Source: CAD feature listing. Evaluate the final solid. Frame: model axes, mm. Face numbers are marked on the shaded views. A direction names the side the tool comes from. Coordinates: 2 decimals unless noted, no trailing zeros. Loops run counter-clockwise (first coordinate to the right, second up) from the corner with the lowest first, then second, coordinate; pieces in that order, holes last. Notation, with made-up numbers: (3, 12.25) - (9, 12.25) arc R20 cw to (9, 39.25) - close; hole circle Ø5 at (50, 7). An arc over 180 degrees is marked (long way). Use CSV: the item, a comma, the result in double quotes. Start each with the question number.
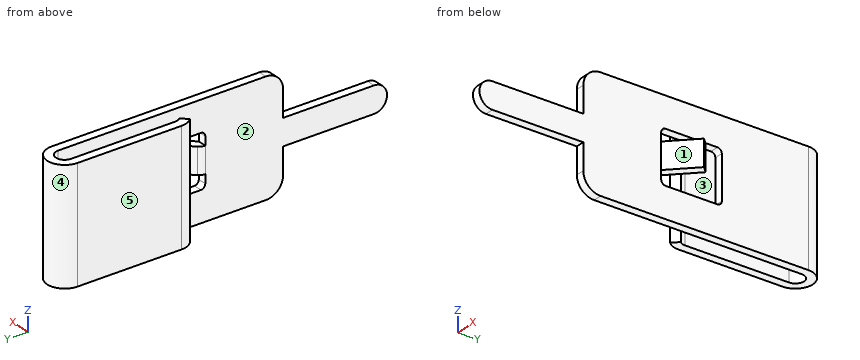
```python
from build123d import *

# Parameters (mm, degrees)
EXTRUDE_1_DEPTH     = 6.5
CUT_EXTRUDE_1_DEPTH = 2
SKETCH_3_W          = 2
SKETCH_3_H          = 2
CUT_EXTRUDE_2_DEPTH = 2.5
SKETCH_4_W          = 2
SKETCH_4_H          = 2
CUT_EXTRUDE_3_DEPTH = 2.5
CUT_EXTRUDE_4_DEPTH = 0.6
SKETCH_6_W          = 1.5
SKETCH_6_H          = 0.707106781
EXTRUDE_2_DEPTH     = 0.5
CUT_EXTRUDE_5_DEPTH = 2
FILLET_1_R          = 0.5


with BuildPart() as part:
    # Эскиз1 → Бобышка-Вытянуть1 (new body)
    with BuildSketch(Plane.XY):
        with BuildLine():
            Line((-2, 19), (-2, 13))
            ThreePointArc((-2, 13), (-1.923879533, 12.617316568), (-1.707106781, 12.292893219))
            Line((-1.707106781, 12.292893219), (-1.353553391, 12.646446609))
            ThreePointArc((-1.353553391, 12.646446609), (-1.461939766, 12.808658284), (-1.5, 13))
            Line((-1.5, 13), (-1.5, 19))
            ThreePointArc((-1.5, 19), (-1, 19.5), (-0.5, 19))
            Line((-0.5, 19), (-0.5, 0))
            Line((-0.5, 0), (0, 0))
            Line((0, 0), (0, 10.5))
            Line((0, 10.5), (1.414213562, 11.914213562))
            Line((1.414213562, 11.914213562), (1.060660172, 12.267766953))
            Line((1.060660172, 12.267766953), (0, 11.207106781))
            Line((0, 11.207106781), (0, 19))
            ThreePointArc((0, 19), (-1, 20), (-2, 19))
        make_face()
    extrude(amount=EXTRUDE_1_DEPTH)

    # Эскиз2 → Вырез-Вытянуть1 (cut)
    with BuildSketch(Plane.ZY.offset(0.5)):
        with BuildLine():
            Line((4, 6), (5.5, 6))
            ThreePointArc((5.5, 6), (6.207106781, 6.292893219), (6.5, 7))
            Line((6.5, 7), (8.5, 7))
            Line((8.5, 7), (8.5, -1))
            Line((8.5, -1), (-2, -1))
            Line((-2, -1), (-2, 7))
            Line((-2, 7), (0, 7))
            ThreePointArc((0, 7), (0.292893219, 6.292893219), (1, 6))
            Line((1, 6), (2.5, 6))
            Line((2.5, 6), (2.5, 0.75))
            ThreePointArc((2.5, 0.75), (3.25, 0), (4, 0.75))
            Line((4, 0.75), (4, 6))
        make_face()
    extrude(amount=-CUT_EXTRUDE_1_DEPTH, mode=Mode.SUBTRACT)

    # Эскиз3 → Вырез-Вытянуть2 (cut)
    with BuildSketch(Plane.XY.offset(6.5)):
        with Locations((1, 11.5)):
            Rectangle(SKETCH_3_W, SKETCH_3_H)
    extrude(amount=-CUT_EXTRUDE_2_DEPTH, mode=Mode.SUBTRACT)

    # Эскиз4 → Вырез-Вытянуть3 (cut)
    with BuildSketch(Plane(origin=(0, 0, 0), x_dir=(-1, 0, 0), z_dir=(0, 0, -1))):
        with Locations((-1, 11.5)):
            Rectangle(SKETCH_4_W, SKETCH_4_H)
    extrude(amount=-CUT_EXTRUDE_3_DEPTH, mode=Mode.SUBTRACT)

    # Эскиз5 → Вырез-Вытянуть4 (cut)
    with BuildSketch(Plane(origin=(0, 0, 0), x_dir=(0, 0, -1), z_dir=(1, 0, 0))):
        with BuildLine():
            Line((-3.25, 10.5), (-2, 10.5))
            ThreePointArc((-2, 10.5), (-1.823223305, 10.573223305), (-1.75, 10.75))
            Line((-1.75, 10.75), (-1.75, 13.75))
            ThreePointArc((-1.75, 13.75), (-1.823223305, 13.926776695), (-2, 14))
            Line((-2, 14), (-4.5, 14))
            ThreePointArc((-4.5, 14), (-4.676776695, 13.926776695), (-4.75, 13.75))
            Line((-4.75, 13.75), (-4.75, 10.75))
            ThreePointArc((-4.75, 10.75), (-4.676776695, 10.573223305), (-4.5, 10.5))
            Line((-4.5, 10.5), (-3.25, 10.5))
        make_face()
    extrude(amount=-CUT_EXTRUDE_4_DEPTH, mode=Mode.SUBTRACT)

    # Эскиз6 → Бобышка-Вытянуть2 (add)
    with BuildSketch(Plane.ZY):
        with Locations((3.25, 10.853553391)):
            Rectangle(SKETCH_6_W, SKETCH_6_H)
    extrude(amount=EXTRUDE_2_DEPTH)

    # Эскиз7 → Вырез-Вытянуть5 (cut)
    with BuildSketch(Plane(origin=(0, 0, 2.5), x_dir=(-1, 0, 0), z_dir=(0, 0, -1))):
        Polygon((0, 11.207106781), (0.5, 10.707106781), (1, 10.707106781), (1, 11.207106781), align=None)
    extrude(amount=-CUT_EXTRUDE_5_DEPTH, mode=Mode.SUBTRACT)

    # Скругление1
    fillet_1_edges = [part.edges().sort_by_distance(p)[0] for p in [
        (-0.5, 10.707106781, 3.25),
    ]]
    fillet(fillet_1_edges, radius=FILLET_1_R)


solid = part.part
```
(1) Draft query along Y for the marked faces 3, 4 and 5. Return one class per face: released by +Y, released by -Y, zero draft, split by the parting line, or undercut.
(2) Section D-D on x = -1. Output: boundary loops of the cut face in (y, z), plus the area to 3 significant figures.
(3) Reachability of the marked faces 1 and 2 from +Z, -Z, +X, -X, +Y, -Y: full face, straight path, thin tool, end or side. Return the list, or none.
(4) Section B-B on y = 16.75. Output: boundary loops of the cut face in (x, z).
(5) Section C-C on z = 4.25. Output: boundary loops of the cut face in (x, y), plus the area to 3 significant figures.
(6) Ray query, line 1 (Z direction, x = -0.4, y = 12); line 2 (X direction, y = 18.5, z = 3.25); line 3 (X direction, y = 7, z = 4.25). Return the intervals inside material, ascending. Write a range as [from, to].
(7) Pin query (flat end, axial travel): pin 1 Ø0.6 at (x, y) = (0, 2.5) entering from +Z; pin 2 Ø3 at (y, z) = (14, 4.5) entering from +X; pin 3 Ø0.6 at (x, z) = (-0.5, 2) entering from -Y. Return the tip coordinate at first contact, or that it passes through.
(8) Section A-A on z = 3.25. Output: boundary loops of the cut face in (x, y).
Solution:
1,face 3,"undercut"
1,face 4,"released by +Y"
1,face 5,"zero draft"
2,outline,"(19.5, 0) - (20, 0) - (20, 6.5) - (19.5, 6.5) - close"
2,area,"3.25 mm²"
3,face 1,"+Z, -Z, +X, -Y"
3,face 2,"+Z, -Z, -Y"
4,outline,"(-2, 0) - (-1.5, 0) - (-1.5, 6.5) - (-2, 6.5) - close; (-0.5, 0) - (0, 0) - (0, 6.5) - (-0.5, 6.5) - close"
5,outline,"(-2, 13) arc R1 ccw to (-1.71, 12.29) - (-1.35, 12.65) arc R0.5 cw to (-1.5, 13) - (-1.5, 19) arc R0.5 cw to (-0.5, 19) - (-0.5, 14) - (0, 14) - (0, 19) arc R1 ccw to (-2, 19) - close; (-0.5, 6) - (0, 6) - (0, 10.5) - (-0.5, 10.5) - close"
5,area,"9.22 mm²"
6,line 1,"z = [0, 1.75], [4.75, 6.5]"
6,line 2,"x = [-2, -1.5], [-0.5, 0]"
6,line 3,"x = [-0.5, 0]"
7,pin 1,"stops at z = 4"
7,pin 2,"stops at x = 0"
7,pin 3,"stops at y = 6"
8,outline,"(-2, 13) arc R1 ccw to (-1.71, 12.29) - (-1.35, 12.65) arc R0.5 cw to (-1.5, 13) - (-1.5, 19) arc R0.5 cw to (-0.5, 19) - (-0.5, 14) - (0, 14) - (0, 19) arc R1 ccw to (-2, 19) - close; (-0.5, 0) - (0, 0) - (0, 10.5) - (1.41, 11.91) - (1.06, 12.27) - (-0.35, 10.85) arc R0.5 ccw to (-0.5, 10.5) - close"
